The listing builds one solid part. Answer for the finished solid, in the listing's coordinates (mm). Face numbers are marked on the shaded views. Give positions to 0.01 mm unless a question says otherwise; leave off trailing zeros. Loops run counter-clockwise (first coordinate to the right, second up) from the corner with the lowest first, then second, coordinate; pieces in that order, holes last. Notation, with made-up numbers: M 28.25,64 L 57.25,64 A20 ccw 57.25,73 Z; hole C 0.5,75.25 d7. An arc over 180 degrees is marked long. Return JSON: item names as keys, results as strings.
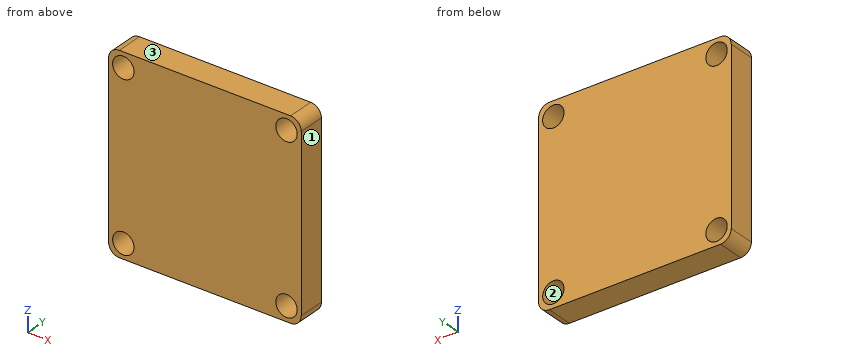
Autodesk Inventor part; units mm, degrees
ref_plane "YZ Plane" through (0, 0, 0) normal (1, 0, 0) x (0, 1, 0)
ref_plane "XZ Plane" through (0, 0, 0) normal (0, 1, 0) x (-1, 0, 0)
ref_plane "XY Plane" through (0, 0, 0) normal (0, 0, 1) x (1, 0, 0)
sketch "Sketch1" plane through (0, 0, 0) normal (0, 1, 0) x (-1, 0, 0)
  line L0 (0, 0) -> (18, 0)
  line L1 (16, -18) -> (-16, -18)
  line L2 (-18, -16) -> (-18, 16)
  line L3 (-16, 18) -> (16, 18)
  line L4 (18, 16) -> (18, -16)
  circle A0 centre (15.25, 15.25) radius 2
  circle A1 centre (-15.25, 15.25) radius 2
  circle A2 centre (-15.25, -15.25) radius 2
  circle A3 centre (15.25, -15.25) radius 2
  arc A4 (16, -18) -> (18, -16) centre (16, -16) ccw
  arc A5 (18, 16) -> (16, 18) centre (16, 16) ccw
  arc A6 (-16, 18) -> (-18, 16) centre (-16, 16) ccw
  arc A7 (-18, -16) -> (-16, -18) centre (-16, -16) ccw
  point P0 (18, -18)
  point P1 (-18, 18)
  point P2 (-18, -18)
  point P3 (18, 18)
  dimension "d0" = 18
  dimension "d1" = 18
  dimension "d2" = 36
  dimension "d3" = 36
  dimension "d6" = 30.5
  dimension "d7" = 30.5
  dimension "d8" = 15.25
  dimension "d9" = 2.75
  dimension "d10" = 4
  dimension "d11" = 4
  dimension "d12" = 4
  dimension "d13" = 4
  dimension "d14" = 2
  dimension "d15" = 2
extrude "Extrusion2" add sketch "Sketch1" along normal blind 5
properties part number "Flight_controler"
(1) Straight lines are drawn through the part: line 1 along Z through (x, y) = (-15.25, 1.1); line 2 along X through (y, z) = (4, 16). For each, find the intervals that lie inside material, in ascending order.
Values follow:
{"line 1": "-18 to -17.25, -13.25 to 13.25, 17.25 to 18", "line 2": "-18 to -17.1, -13.4 to 13.4, 17.1 to 18"}
(2) The part is cut by section B-B (x = 15.25). Determine the outline of the cut face in (y, z).
Values follow:
{"outline": "M 0,-18 L 5,-18 L 5,-17.25 L 0,-17.25 Z; M 0,-13.25 L 5,-13.25 L 5,13.25 L 0,13.25 Z; M 0,17.25 L 5,17.25 L 5,18 L 0,18 Z"}
(3) The part is cut by section A-A (z = -15.25). Determine the outline of the cut face in (x, y), and give its area (3 significant figures).
Values follow:
{"outline": "M -18,0 L -17.25,0 L -17.25,5 L -18,5 Z; M -13.25,0 L 13.25,0 L 13.25,5 L -13.25,5 Z; M 17.25,0 L 18,0 L 18,5 L 17.25,5 Z", "area": "140 mm²"}
(4) The part is cut by section C-C (y = 1.2). Determine the outline of the cut face in (x, z).
Values follow:
{"outline": "M -18,-16 A2 ccw -16,-18 L 16,-18 A2 ccw 18,-16 L 18,16 A2 ccw 16,18 L -16,18 A2 ccw -18,16 Z; hole C -15.25,-15.25 d4; hole C -15.25,15.25 d4; hole C 15.25,-15.25 d4; hole C 15.25,15.25 d4"}
(5) Determine the mould class of the marked faces 1, 2 and 3 for opening direction X: released by +X, released by -X, zero draft, split by the parting line, or undercut.
Values follow:
{"face 1": "released by +X", "face 2": "undercut", "face 3": "zero draft"}
(6) Given pin 1 (3 mm diameter, centred on x = 15.25, z = 15.25, fed in from +Y), flat-ended and moving along its own axis, determine where the tip first touches the part or whether it passes through.
Values follow:
{"pin 1": "through"}
